from build123d import *

# Parameters (mm, degrees)
SKETCH1_W           = 15
SKETCH1_H           = 15
BOSS_EXTRUDE1_DEPTH = 15
BOSS_EXTRUDE2_DEPTH = 5
SKETCH7_R           = 2.5
CUT_EXTRUDE1_DEPTH  = 4
SKETCH13_R          = 2.5
CUT_EXTRUDE6_DEPTH  = 4
SKETCH16_R          = 2.5
CUT_EXTRUDE7_DEPTH  = 4
CHAMFER1_SIZE       = 1


with BuildPart() as part:
    # Sketch1 → Boss-Extrude1 (new body)
    with BuildSketch(Plane.XY):
        with Locations((7.5, 7.5)):
            Rectangle(SKETCH1_W, SKETCH1_H)
    extrude(amount=BOSS_EXTRUDE1_DEPTH)

    # Sketch2 → Boss-Extrude2 (add)
    with BuildSketch(Plane.XY.offset(15)):
        with BuildLine():
            ThreePointArc((9.232411614, 9.232411614), (5.767588386, 9.232411614), (5.767588386, 5.767588386))
            Line((5.767588386, 5.767588386), (9.232411614, 9.232411614))
        make_face()
        with BuildLine():
            Line((9.232411614, 9.232411614), (5.767588386, 5.767588386))
            ThreePointArc((5.767588386, 5.767588386), (8.437574409, 5.236495145), (9.95, 7.5))
            ThreePointArc((9.95, 7.5), (9.763504855, 8.437574409), (9.232411614, 9.232411614))
        make_face()
    extrude(amount=BOSS_EXTRUDE2_DEPTH)

    # Sketch7 → Cut-Extrude1 (cut)
    with BuildSketch(Plane.ZY):
        with Locations((7.5, 7.5)):
            Circle(SKETCH7_R)
    extrude(amount=-CUT_EXTRUDE1_DEPTH, mode=Mode.SUBTRACT)

    # Sketch13 → Cut-Extrude6 (cut)
    with BuildSketch(Plane(origin=(0, 15, 0), x_dir=(1, 0, 0), z_dir=(0, 1, 0))):
        with Locations(Location((7.5, -7.5, 0), (0, 0, 270))):
            Circle(SKETCH13_R)
    extrude(amount=-CUT_EXTRUDE6_DEPTH, mode=Mode.SUBTRACT)

    # Sketch16 → Cut-Extrude7 (cut)
    with BuildSketch(Plane(origin=(0, 0, 0), x_dir=(-1, 0, 0), z_dir=(0, 0, -1))):
        with Locations((-7.5, 7.5)):
            Circle(SKETCH16_R)
    extrude(amount=-CUT_EXTRUDE7_DEPTH, mode=Mode.SUBTRACT)

    # Chamfer1
    chamfer1_edges = [part.edges().sort_by_distance(p)[0] for p in [
        (15, 7.5, 15),
        (7.5, 15, 15),
        (0, 7.5, 15),
        (7.5, 15, 0),
        (15, 7.5, 0),
        (7.5, 0, 0),
        (0, 7.5, 0),
        (0, 15, 7.5),
        (15, 15, 7.5),
        (15, 0, 7.5),
        (0, 0, 7.5),
        (7.5, 0, 15),
    ]]
    chamfer(chamfer1_edges, length=CHAMFER1_SIZE)

    # Fillet1: read off the stored shape, not the designer's step
    # Fillet1 outline → Fillet1 (revolve, cut)
    with BuildSketch(Plane(origin=(7.5, 7.5, 0), x_dir=(1, 0, 0), z_dir=(0, -1, 0))):
        with BuildLine():
            ThreePointArc((1.95, 20), (2.303553391, 19.853553391), (2.45, 19.5))
            Line((2.45, 19.5), (2.45, 20))
            Line((2.45, 20), (1.95, 20))
        make_face()
        with BuildLine():
            ThreePointArc((3, 0), (2.646446609, 0.146446609), (2.5, 0.5))
            Line((2.5, 0.5), (2.5, 0))
            Line((2.5, 0), (3, 0))
        make_face()
    revolve(axis=Axis((7.5, 7.5, 0), (0, 0, 1)), mode=Mode.SUBTRACT)

    # Fillet1 2 outline → Fillet1 2 (revolve, cut)
    with BuildSketch(Plane(origin=(7.5, 0, 7.5), x_dir=(1, 0, 0), z_dir=(0, 0, 1))):
        with BuildLine():
            Line((2.5, 15), (2.5, 14.5))
            ThreePointArc((2.5, 14.5), (2.646446609, 14.853553391), (3, 15))
            Line((3, 15), (2.5, 15))
        make_face()
    revolve(axis=Axis((7.5, 0, 7.5), (0, 1, 0)), mode=Mode.SUBTRACT)

    # Fillet1 3 outline → Fillet1 3 (revolve, cut)
    with BuildSketch(Plane(origin=(0, 7.5, 7.5), x_dir=(0, 1, 0), z_dir=(0, 0, -1))):
        with BuildLine():
            ThreePointArc((3, 0), (2.646446609, 0.146446609), (2.5, 0.5))
            Line((2.5, 0.5), (2.5, 0))
            Line((2.5, 0), (3, 0))
        make_face()
    revolve(axis=Axis((0, 7.5, 7.5), (1, 0, 0)), mode=Mode.SUBTRACT)


solid = part.part
Here's how the part is built. I have some questions about the finished solid (model axes, mm). A direction names the side the tool comes from. Give positions to 0.01 mm unless a question says otherwise; leave off trailing zeros. Write each loop counter-clockwise with the first axis right and the second up, starting at its lowest first coordinate (ties: lowest second). Pieces come first, ordered by that corner, then holes. Notation, with made-up numbers: (68.5, -28) -> (116.5, -28) arc R27 ccw to (116.5, 2) -> close; hole circle Ø8 at (16, -28). An arc over 180 degrees is marked (long way). Use one line per item in the form item = value. Start each with the question number.
1. Thinking about a two-plate mould opening in X: for faces 1 (the face through (14.5, 7.4, 14.5)), 2 (the face through (0, 10.3, 6)), 3 (the face through (8, 8, 4)), 4 (the face through (8.04, 5.06, 2.23)), which applies, +X half, -X half, draft (parallel to the pull), parting line (faces both ways), or undercut?
2. Imagine slicing it at A-A on z = 2. List the corners of the cut face in (x, y) for me.
3. Will these pins go through, and if not, where does the flat tip stop? pin 1 Ø1.5 at (x, y) = (2, 5.5) entering from +Z; pin 2 Ø1 at (x, z) = (11.5, 15) entering from -Y; pin 3 Ø1.5 at (y, z) = (7.5, 7) entering from -X.
4. On a 3-axis mill with a long thin cutter (end or side, diameter ignored), from which of +Z, -Z, +X, -X, +Y, -Y can I reach the whole of each face in a straight line? I mean faces 5 (the face through (0.5, 7.4, 14.5)), 6 (the face through (10.3, 7.6, 15)), 7 (the face through (2.23, 5.28, 8.65)). Say none if no direction works.
5. If I drill on L1, parallel to Y at x = 2.95, z = 7.5; L2, parallel to Y at x = 7, z = 2.25, over which ranges is the centre line in solid material (lowest first)?
6. Imagine slicing it at B-B on x = 12. List the corners of the cut face in (y, z) for me, plus the area to 3 significant figures.
7. Imagine slicing it at D-D on z = 7.5. List the corners of the cut face in (x, y) for me, plus the area to 3 significant figures.
Entries:
q1.face_1 = +X half
q1.face_2 = -X half
q1.face_3 = undercut
q1.face_4 = undercut
q2.outline = (0, 1) -> (1, 0) -> (14, 0) -> (15, 1) -> (15, 14) -> (14, 15) -> (1, 15) -> (0, 14) -> close; hole circle Ø5 at (7.5, 7.5)
q3.pin_1 = 15
q3.pin_2 = 0.5
q3.pin_3 = 4
q4.face_5 = +Z, -X, +Y, -Y
q4.face_6 = +Z
q4.face_7 = -X
q5.L1 = 0 to 5, 10 to 15
q5.L2 = 0 to 5.05, 9.95 to 15
q6.outline = (0, 1) -> (1, 0) -> (14, 0) -> (15, 1) -> (15, 14) -> (14, 15) -> (1, 15) -> (0, 14) -> close
q6.area = 223 mm²
q7.outline = (0, 1) -> (1, 0) -> (14, 0) -> (15, 1) -> (15, 14) -> (14, 15) -> (10.5, 15) arc R0.5 ccw to (10, 14.5) -> (10, 11) -> (5, 11) -> (5, 14.5) arc R0.5 ccw to (4.5, 15) -> (1, 15) -> (0, 14) -> (0, 10.5) arc R0.5 ccw to (0.5, 10) -> (4, 10) -> (4, 5) -> (0.5, 5) arc R0.5 ccw to (0, 4.5) -> close
q7.area = 183 mm²
